Read the model definition and answer for the solid it produces. Units are mm, in the model's axes. A direction names the side the tool comes from. Give positions to 0.01 mm unless a question says otherwise; leave off trailing zeros. Order: outer loops, then holes, each group sorted by start corner. A loop starts at its lowest first (then second) coordinate and runs counter-clockwise, first axis right, second up.
```python
from build123d import *

# Parameters (mm, degrees)
CROQUIS1_R              = 11.025
SALIENTE_EXTRUIR1_DEPTH = 5
CROQUIS2_W              = 90
CROQUIS2_H              = 5
SALIENTE_EXTRUIR2_DEPTH = 90
CROQUIS3_R              = 21.5
SALIENTE_EXTRUIR3_DEPTH = 50
CROQUIS4_R              = 2.5
CORTAR_EXTRUIR1_DEPTH   = 70
CROQUIS5_R              = 2.5
CORTAR_EXTRUIR2_DEPTH   = 130.131715701


with BuildPart() as part:
    # Croquis1 → Saliente-Extruir1 (new body)
    with BuildSketch(Plane.XY):
        with BuildLine():
            Line((45, -2.305306559), (45, -35))
            Line((45, -35), (-45, -35))
            Line((-45, -35), (-45, 25))
            ThreePointArc((-45, 25), (-39.142135624, 39.142135624), (-25, 45))
            Line((-25, 45), (25, 45))
            ThreePointArc((25, 45), (39.142135624, 39.142135624), (45, 25))
            Line((45, 25), (45, -2.305306559))
        make_face()
        Circle(CROQUIS1_R, mode=Mode.SUBTRACT)
    extrude(amount=-SALIENTE_EXTRUIR1_DEPTH)

    # Croquis2 → Saliente-Extruir2 (add)
    with BuildSketch(Plane(origin=(0, 0, -5), x_dir=(-1, 0, 0), z_dir=(0, 0, -1))):
        with Locations((0, -32.5)):
            Rectangle(CROQUIS2_W, CROQUIS2_H)
    extrude(amount=SALIENTE_EXTRUIR2_DEPTH)

    # Croquis3 → Saliente-Extruir3 (add)
    with BuildSketch(Plane(origin=(0, 0, -5), x_dir=(-1, 0, 0), z_dir=(0, 0, -1))):
        with BuildLine():
            Line((17, -30), (17, -19.672315573))
            ThreePointArc((17, -19.672315573), (0, 26), (-17, -19.672315573))
            Line((-17, -19.672315573), (-17, -30))
            Line((-17, -30), (17, -30))
        make_face()
        Circle(CROQUIS3_R, mode=Mode.SUBTRACT)
    extrude(amount=SALIENTE_EXTRUIR3_DEPTH)

    # Croquis4 → Cortar-Extruir1 (cut)
    with BuildSketch(Plane.XY):
        with Locations((-16, 0)):
            Circle(CROQUIS4_R)
        with Locations((16, 0)):
            Circle(CROQUIS4_R)
    extrude(amount=-CORTAR_EXTRUIR1_DEPTH, mode=Mode.SUBTRACT)

    # Croquis5 → Cortar-Extruir2 (cut, through all)
    with BuildSketch(Plane(origin=(0, -30, 0), x_dir=(1, 0, 0), z_dir=(0, 1, 0))):
        with Locations(Location((-35, 85, 0), (0, 0, 180))):
            Circle(CROQUIS5_R)
        with Locations((35, 85)):
            Circle(CROQUIS5_R)
        with Locations(Location((35, 15, 0), (0, 0, 180))):
            Circle(CROQUIS5_R)
        with Locations((-35, 15)):
            Circle(CROQUIS5_R)
    extrude(amount=-CORTAR_EXTRUIR2_DEPTH, mode=Mode.SUBTRACT)


solid = part.part
```
1) A tool of negligible diameter and unlimited length cuts with its end or side. For faces 5 (the face through (0, 45, -2)), 6 (the face through (8, -21, -55)), 7 (the face through (1, -30, -59)), 8 (the face through (1, -35, -47)), 9 (the face through (-17, -25, -30)), from which of +Z, -Z, +X, -X, +Y, -Y can it reach the whole face along a straight path? Write none if from no direction.
Final values:
face 5: +Z, -Z, +X, -X, +Y
face 6: -Z, +X, -X, +Y
face 7: -Z
face 8: +Z, -Z, +X, -X, -Y
face 9: -Z, -X
2) Given pin 1 (6.5 mm diameter, centred on x = 35, z = -15, fed in from +Y); pin 2 (21.5 mm diameter, centred on x = -1.5, y = 5.5, fed in from -Z); pin 3 (12 mm diameter, centred on y = -18.5, z = -20, fed in from -X), each flat-ended and moving along its own axis, determine where each tip first touches the part or whether it passes through.
Final values:
pin 1: stops at y = -30
pin 2: stops at z = -5
pin 3: stops at x = -22.8
3) The part is cut by section D-D on z = -85. Determine the outline of the cut face in (x, y).
Final values:
outline: (-45, -35) - (-37.5, -35) - (-37.5, -30) - (-45, -30) - close; (-32.5, -35) - (32.5, -35) - (32.5, -30) - (-32.5, -30) - close; (37.5, -35) - (45, -35) - (45, -30) - (37.5, -30) - close
4) The part is cut by section C-C on x = 35. Determine the outline of the cut face in (y, z).
Final values:
outline: (-35, -95) - (-30, -95) - (-30, -87.5) - (-35, -87.5) - close; (-35, -82.5) - (-30, -82.5) - (-30, -17.5) - (-35, -17.5) - close; (-35, -12.5) - (-30, -12.5) - (-30, -5) - (42.32, -5) - (42.32, 0) - (-35, 0) - close
5) The part is cut by section B-B on y = 0. Determine the outline of the cut face in (x, z) (3 decimals).
Final values:
outline: (-45, -5) - (-26, -5) - (-26, -55) - (-21.5, -55) - (-21.5, -5) - (-18.5, -5) - (-18.5, 0) - (-45, 0) - close; (-13.5, -5) - (-11.025, -5) - (-11.025, 0) - (-13.5, 0) - close; (11.025, -5) - (13.5, -5) - (13.5, 0) - (11.025, 0) - close; (18.5, -5) - (21.5, -5) - (21.5, -55) - (26, -55) - (26, -5) - (45, -5) - (45, 0) - (18.5, 0) - close
6) Consider L1, parallel to Z at x = -35, y = -33; L2, parallel to Y at x = -20, z = -85.5; L3, parallel to Z at x = 25, y = 1. Determine where each line is inside the solid, lowest interval first.
Final values:
L1: z = -95 to -87.5, -82.5 to -17.5, -12.5 to 0
L2: y = -35 to -30
L3: z = -55 to 0
7) The part is cut by section A-A on z = -15. Determine the outline of the cut face in (x, y), and give its area (3 significant figures).
Final values:
outline: (-45, -35) - (-37.5, -35) - (-37.5, -30) - (-45, -30) - close; (-32.5, -35) - (32.5, -35) - (32.5, -30) - (17, -30) - (17, -19.67) arc R26 ccw (long way) to (-17, -19.67) - (-17, -30) - (-32.5, -30) - close; (37.5, -35) - (45, -35) - (45, -30) - (37.5, -30) - close; hole circle Ø43 at (0, 0)
area: 1,280 mm2
8) For a pull along X with two mould halves and no side action, classify faces 1 (the face through (32.69, -32.47, -15.96)), 2 (the face through (17, -25, -30)), 3 (the face through (11, 25, -5)), 4 (the face through (-45, -32, -33)) as released by +X, released by -X, zero draft, split by the parting line, or undercut.
Final values:
face 1: undercut
face 2: released by +X
face 3: zero draft
face 4: released by -X
